The figure shows three views and two pictorial views of one solid part (mm, origin at its lowest corner). Answer the questions. A direction names the side the tool comes from. Round coordinates to 2 decimals unless told otherwise and drop trailing zeros. Loops run counter-clockwise (first coordinate to the right, second up) from the corner with the lowest first, then second, coordinate; pieces in that order, holes last. Notation, with made-up numbers: (31.5, -38) - (78.5, -38) arc R28 ccw to (78.5, -3) - close; hole circle Ø5 at (24.25, -19). An arc over 180 degrees is marked (long way). Use one line per item in the form item = value. Start each with the question number.
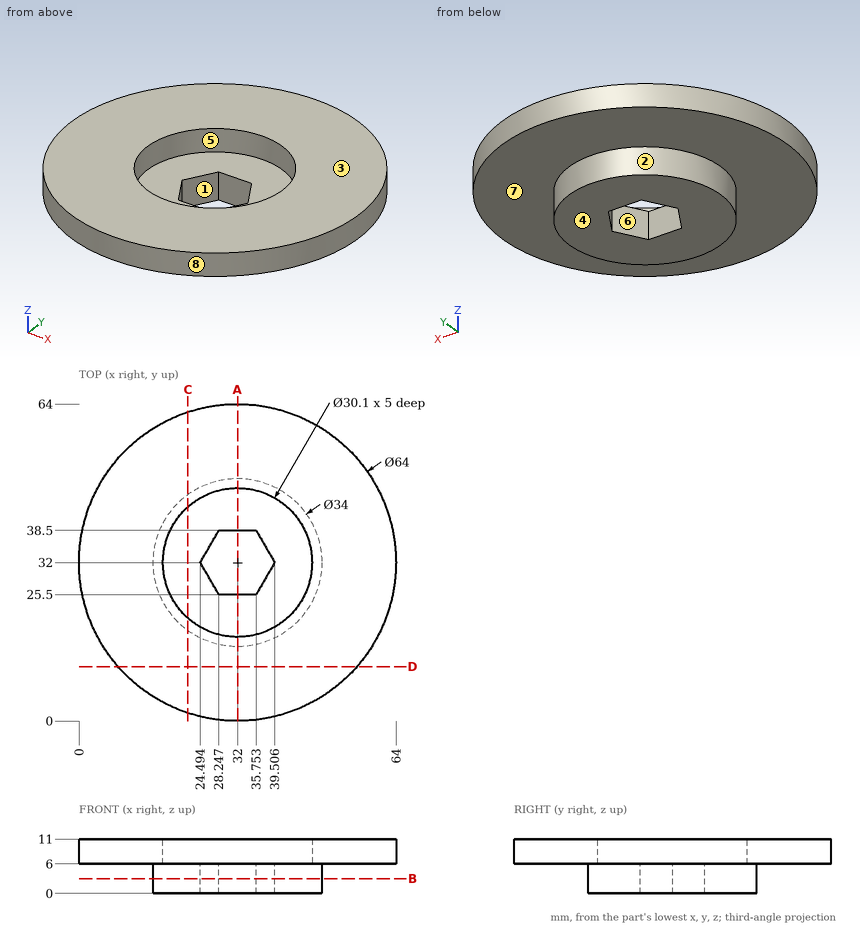
1) A cutting plane is placed at D-D on y = 11. Write down the section's boundary in (x, z) (1 decimal).
2) For the marked faces 1, 2, 3, 4 and 5, determine the directions among +Z, -Z, +X, -X, +Y, -Y from which every point of the face is accessible in a straight line to the end or side of a thin tool.
3) Straight lines are drawn through the part: line 1 (X direction, y = 32, z = 8.25); line 2 (Z direction, x = 24, y = 38). For each, find the intervals that lie inside material, in ascending order. Write a range as from..to.
4) Flat-ended cylindrical pins translate along their axes: pin 1 (4 mm diameter, centred on x = 18, z = 8.5, fed in from +Y) (1 decimal); pin 2 (5 mm diameter, centred on x = 57, z = 6.5, fed in from +Y) (1 decimal); pin 3 (6.5 mm diameter, centred on x = 31, z = 4.5, fed in from +Y). Find the tip coordinate at first contact, or state that the pin passes through.
5) A cutting plane is placed at C-C on x = 22. Write down the section's boundary in (y, z).
6) A cutting plane is placed at B-B on z = 3. Write down the section's boundary in (x, y) (1 decimal).
7) A cutting plane is placed at A-A on x = 32. Write down the section's boundary in (y, z).
8) Determine the mould class of the marked faces 6, 7 and 8 for opening direction Y: +Y half, -Y half, draft (parallel to the pull), parting line (faces both ways), or undercut.
Checks:
q1.outline = (7.9, 6) - (56.1, 6) - (56.1, 11) - (7.9, 11) - close
q2.face_1 = +Z, -Z
q2.face_2 = -Z
q2.face_3 = +Z, +X, -X, +Y, -Y
q2.face_4 = -Z, +X, -X, +Y, -Y
q2.face_5 = +Z
q3.line_1 = 0..16.95, 47.05..64
q3.line_2 = 0..6
q4.pin_1 = 61.7
q4.pin_2 = 54.8
q4.pin_3 = 64
q5.outline = (1.6, 6) - (18.25, 6) - (18.25, 0) - (45.75, 0) - (45.75, 6) - (62.4, 6) - (62.4, 11) - (43.25, 11) - (43.25, 6) - (20.75, 6) - (20.75, 11) - (1.6, 11) - close
q6.outline = circle Ø34 at (32, 32); hole (24.5, 32) - (28.2, 25.5) - (35.8, 25.5) - (39.5, 32) - (35.8, 38.5) - (28.2, 38.5) - close
q7.outline = (0, 6) - (15, 6) - (15, 0) - (25.5, 0) - (25.5, 6) - (16.95, 6) - (16.95, 11) - (0, 11) - close; (38.5, 0) - (49, 0) - (49, 6) - (64, 6) - (64, 11) - (47.05, 11) - (47.05, 6) - (38.5, 6) - close
q8.face_6 = undercut
q8.face_7 = draft
q8.face_8 = parting line
